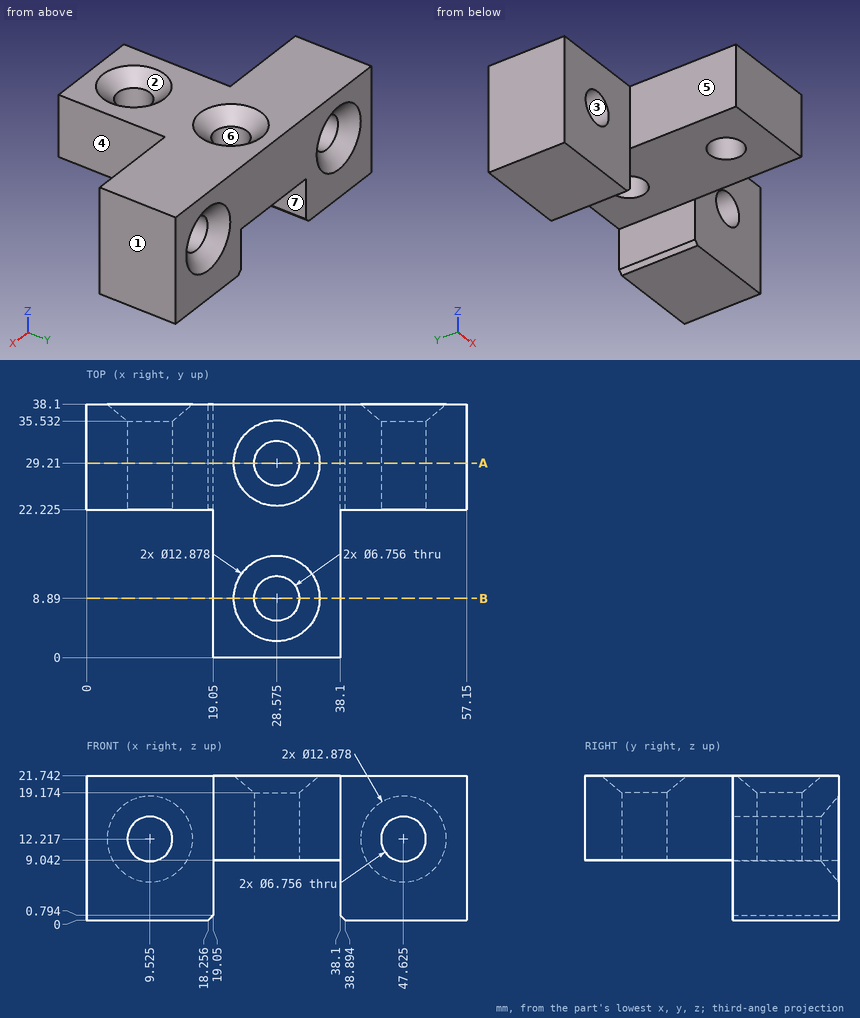
The drawing under review shows one solid part. Ordinate dimensions are in mm from its lowest x, y, z. A direction names the side the tool comes from. Give positions to 0.01 mm unless a question says otherwise; leave off trailing zeros. Loops run counter-clockwise (first coordinate to the right, second up) from the corner with the lowest first, then second, coordinate; pieces in that order, holes last. Notation, with made-up numbers: M 38,10.25 L 92,10.25 A30 cw 92,33.25 Z; hole C -29,44 d8. An arc over 180 degrees is marked long. One line per question, with ' | ' between items. Start each with the question number.
1. To check wall thickness, follow L1, parallel to X at y = 8.89, z = 14.5; L2, parallel to X at y = 34, z = 7; L3, parallel to Y at x = 30, z = 13.25. State the ranges of each line that lie inside material, in increasing order.
2. The part is to be moulded in two halves that separate along Z. For the marked faces 1, 2 and 3, say which applies: released by +Z, released by -Z, zero draft, split by the parting line, or undercut.
3. Add section A-A (y = 29.21). Give the number of separate pieces and of enclosed holes in the cut face.
4. For the marked faces 4, 5, 6 and 7, list the 3-axis set-ups (+Z, -Z, +X, -X, +Y, -Y) from which the entire face can be reached by the end or side of a thin tool; tool diameter is ignored.
5. Insertion check: P1, Ø4, axis at y = 18.5, z = 10, coming from the -X side; P2, Ø9.5, axis at x = 13.5, z = 6.5, coming from the -Y side (3 decimals); P3, Ø9, axis at x = 28.575, y = 29.21, coming from the -Z side. Each pin has a flat end and moves straight along its axis. Give the tip position at first contact, or say it passes through.
6. Add section B-B (y = 8.89). Write out the cut boundary in (x, z).
Worked out:
1) L1: x = 19.05 to 25.2, 31.95 to 38.1 | L2: x = 0 to 19.05, 38.1 to 57.15 | L3: y = 0 to 5.83, 11.95 to 26.15, 32.27 to 38.1
2) face 1: zero draft | face 2: released by +Z | face 3: undercut
3) separate pieces: 2 | enclosed holes: 2
4) face 4: +Z, -Z, +X, -Y | face 5: +Z, -Z, -X, -Y | face 6: +Z, -Z | face 7: -Z, +Y, -Y
5) P1: stops at x = 19.05 | P2: stops at y = 22.225 | P3: stops at z = 9.04
6) outline: M 19.05,9.04 L 25.2,9.04 L 25.2,19.17 L 22.14,21.74 L 19.05,21.74 Z; M 31.95,9.04 L 38.1,9.04 L 38.1,21.74 L 35.01,21.74 L 31.95,19.17 Z
